```python
from build123d import *

# Parameters (mm, degrees)
F0_W     = 152.4
F0_H     = 76.2
F0_R     = 8.89
F1_DEPTH = 25.4
F2_W     = 25.4
F2_H     = 50.8


with BuildPart() as f1:
    # F0 (on Top) → F1 (new body)
    with BuildSketch(Plane.XY):
        Rectangle(F0_W, F0_H)
        with Locations((-66.770934, -26.765937)):
            Circle(F0_R, mode=Mode.SUBTRACT)
        with Locations((59.575796, -23.887878)):
            Circle(F0_R, mode=Mode.SUBTRACT)
        with Locations((-64.756297, 26.190324)):
            Circle(F0_R, mode=Mode.SUBTRACT)
        with Locations((64.180687, 26.765937)):
            Circle(F0_R, mode=Mode.SUBTRACT)
    extrude(amount=F1_DEPTH)

    # F2 (on Front) → F3 (revolve)
    with BuildSketch(Plane.XZ):
        with Locations((12.7, 50.8)):
            Rectangle(F2_W, F2_H)
    revolve(axis=Axis((0, 0, 50.8), (0, 0, 1)))


solid = f1.part
```
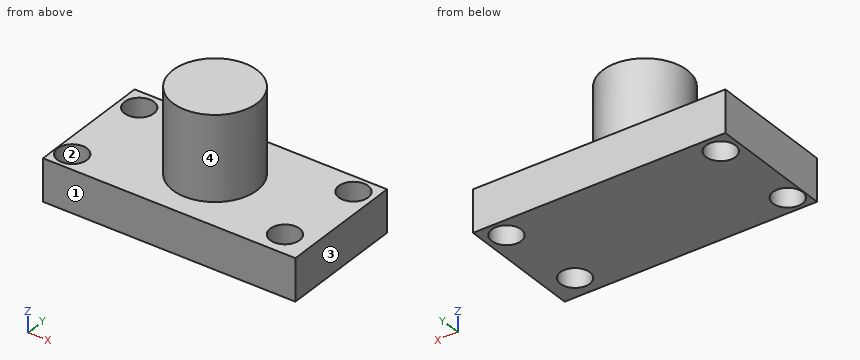
Model file for the job. Use its own axes, mm. Face numbers are marked on the shaded views. Coordinates: 2 decimals unless noted, no trailing zeros. Order: outer loops, then holes, each group sorted by start corner. A loop starts at its lowest first (then second) coordinate and runs counter-clockwise, first axis right, second up. Notation, with made-up numbers: (14.5, 18.25) -> (39.5, 18.25) arc R27 ccw to (39.5, 47.25) -> close; hole circle Ø1 at (0, -36.5). An arc over 180 degrees is marked (long way). Return JSON: item names as keys, results as strings.
Item 1: Mould opens along X. For the marked faces 1, 2, 3 and 4 say: pulls with the +X half, pulls with the -X half, needs draft (parallel to the pull), parting line crosses it, or undercut.
Model answer:
{"face 1": "needs draft", "face 2": "undercut", "face 3": "pulls with the +X half", "face 4": "parting line crosses it"}
Item 2: Slice it at D-D (x = -61.5). Write the cut outline in (y, z).
Model answer:
{"outline": "(-38.1, 0) -> (-33.92, 0) -> (-33.92, 25.4) -> (-38.1, 25.4) -> close; (-19.61, 0) -> (17.92, 0) -> (17.92, 25.4) -> (-19.61, 25.4) -> close; (34.46, 0) -> (38.1, 0) -> (38.1, 25.4) -> (34.46, 25.4) -> close"}
Item 3: Slice it at B-B (x = 0). Write the cut outline in (y, z), then the cut area to 3 significant figures.
Model answer:
{"outline": "(-38.1, 0) -> (38.1, 0) -> (38.1, 25.4) -> (25.4, 25.4) -> (25.4, 76.2) -> (-25.4, 76.2) -> (-25.4, 25.4) -> (-38.1, 25.4) -> close", "area": "4,520 mm²"}
Item 4: Slice it at A-A (y = 0). Write the cut outline in (x, z).
Model answer:
{"outline": "(-76.2, 0) -> (76.2, 0) -> (76.2, 25.4) -> (25.4, 25.4) -> (25.4, 76.2) -> (-25.4, 76.2) -> (-25.4, 25.4) -> (-76.2, 25.4) -> close"}
Item 5: Pin check, flat tips, straight feed: P1, Ø20.5, axis at x = 64.18, y = 26.77, coming from the +Z side; P2, Ø1.5, axis at x = 24, z = 46.5, coming from the +Y side; P3, Ø1, axis at x = 10.5, y = 18, coming from the -Z side; P4, Ø10, axis at y = -22.5, z = 67, coming from the +X side. Stop position of each tip, or through.
Model answer:
{"P1": "stops at z = 25.4", "P2": "stops at y = 10.23", "P3": "stops at z = 0", "P4": "stops at x = 18.41"}
Item 6: Slice it at C-C (y = 21.5). Write the cut outline in (x, z), then the cut area to 3 significant figures.
Model answer:
{"outline": "(-76.2, 0) -> (-72.31, 0) -> (-72.31, 25.4) -> (-76.2, 25.4) -> close; (-57.2, 0) -> (57.02, 0) -> (57.02, 25.4) -> (13.52, 25.4) -> (13.52, 76.2) -> (-13.52, 76.2) -> (-13.52, 25.4) -> (-57.2, 25.4) -> close; (71.34, 0) -> (76.2, 0) -> (76.2, 25.4) -> (71.34, 25.4) -> close", "area": "4,500 mm²"}
Item 7: Wall check: line 1 along X through (y, z) = (26.5, 13); line 2 along Y through (x, z) = (66.5, 10); line 3 along X through (y, z) = (31.5, 14). Give the ranges that are in metal, low to high. Write a range as from..to.
Model answer:
{"line 1": "x = -76.2..-73.64, -55.87..55.29, 73.07..76.2", "line 2": "y = -38.1..-29.46, -18.31..18.18, 35.35..38.1", "line 3": "x = -76.2..-71.89, -57.63..56.66, 71.71..76.2"}
